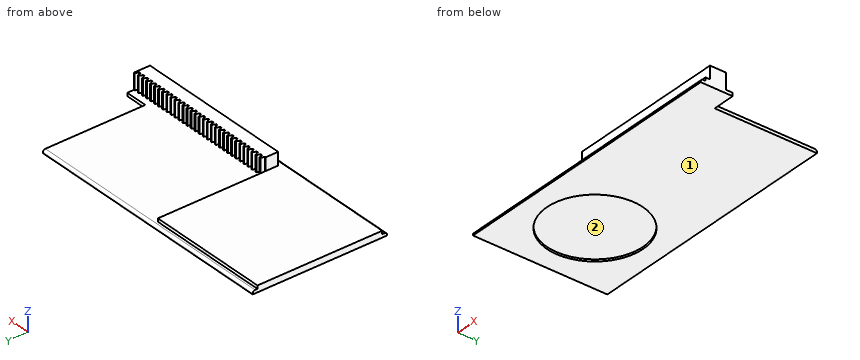
from build123d import *

# Parameters (mm, degrees)
SKETCH1_W           = 206.375
SKETCH1_H           = 106.68
BOSS_EXTRUDE1_DEPTH = 2.54
BOSS_EXTRUDE2_DEPTH = 12.7
SKETCH3_W           = 17.745286293
SKETCH3_H           = 25.4
BOSS_EXTRUDE3_DEPTH = 2.54
FILLET1_R           = 1.905
BOSS_EXTRUDE4_DEPTH = 2.54
SKETCH6_R           = 38.1
CUT_EXTRUDE1_DEPTH  = 1.5875


with BuildPart() as part:
    # Sketch1 → Boss-Extrude1 (new body)
    with BuildSketch(Plane.XY):
        with Locations((49.2125, 0)):
            Rectangle(SKETCH1_W, SKETCH1_H)
    extrude(amount=BOSS_EXTRUDE1_DEPTH)

    # Sketch2 → Boss-Extrude2 (add)
    with BuildSketch(Plane.XY.offset(2.54)):
        Polygon((170.145286293, -33.159030477), (169.379659355, -33.159030477), (168.362726521, -35.953030477), (167.172396462, -35.953030477), (166.155463627, -33.159030477), (165.38983669, -33.159030477), (164.372903855, -35.953030477), (163.182573796, -35.953030477), (162.165640962, -33.159030477), (161.400014024, -33.159030477), (160.38308119, -35.953030477), (159.192751131, -35.953030477), (158.175818296, -33.159030477), (157.410191359, -33.159030477), (156.393258524, -35.953030477), (155.202928465, -35.953030477), (154.185995631, -33.159030477), (153.420368693, -33.159030477), (152.403435859, -35.953030477), (151.2131058, -35.953030477), (150.196172965, -33.159030477), (149.430546028, -33.159030477), (148.413613193, -35.953030477), (147.223283134, -35.953030477), (146.2063503, -33.159030477), (145.440723362, -33.159030477), (144.423790528, -35.953030477), (143.233460469, -35.953030477), (142.216527634, -33.159030477), (141.450900697, -33.159030477), (140.433967862, -35.953030477), (139.243637803, -35.953030477), (138.226704969, -33.159030477), (137.461078031, -33.159030477), (136.444145197, -35.953030477), (135.253815138, -35.953030477), (134.236882303, -33.159030477), (133.471255366, -33.159030477), (132.454322531, -35.953030477), (131.263992472, -35.953030477), (130.247059638, -33.159030477), (129.4814327, -33.159030477), (128.464499866, -35.953030477), (127.274169807, -35.953030477), (126.257236972, -33.159030477), (125.491610035, -33.159030477), (124.4746772, -35.953030477), (123.284347141, -35.953030477), (122.267414307, -33.159030477), (121.501787369, -33.159030477), (120.484854535, -35.953030477), (119.294524476, -35.953030477), (118.277591641, -33.159030477), (117.511964704, -33.159030477), (116.495031869, -35.953030477), (115.30470181, -35.953030477), (114.287768976, -33.159030477), (113.522142038, -33.159030477), (112.505209204, -35.953030477), (111.314879145, -35.953030477), (110.29794631, -33.159030477), (109.532319373, -33.159030477), (108.515386538, -35.953030477), (107.325056479, -35.953030477), (106.308123645, -33.159030477), (105.542496707, -33.159030477), (104.525563873, -35.953030477), (103.335233814, -35.953030477), (102.318300979, -33.159030477), (101.552674042, -33.159030477), (100.535741207, -35.953030477), (99.345411148, -35.953030477), (98.328478314, -33.159030477), (97.562851376, -33.159030477), (96.545918542, -35.953030477), (95.355588483, -35.953030477), (94.338655648, -33.159030477), (93.573028711, -33.159030477), (92.556095876, -35.953030477), (91.365765817, -35.953030477), (90.348832983, -33.159030477), (89.583206045, -33.159030477), (88.566273211, -35.953030477), (87.375943152, -35.953030477), (86.359010317, -33.159030477), (85.59338338, -33.159030477), (84.576450545, -35.953030477), (83.386120486, -35.953030477), (82.369187652, -33.159030477), (81.603560714, -33.159030477), (80.58662788, -35.953030477), (79.396297821, -35.953030477), (78.379364986, -33.159030477), (77.613738049, -33.159030477), (76.596805214, -35.953030477), (75.406475155, -35.953030477), (74.389542321, -33.159030477), (73.623915383, -33.159030477), (72.606982549, -35.953030477), (71.41665249, -35.953030477), (70.399719655, -33.159030477), (69.634092718, -33.159030477), (68.617159883, -35.953030477), (67.426829824, -35.953030477), (66.40989699, -33.159030477), (65.644270052, -33.159030477), (64.627337218, -35.953030477), (63.437007159, -35.953030477), (62.420074324, -33.159030477), (61.654447387, -33.159030477), (60.637514552, -35.953030477), (59.447184493, -35.953030477), (58.430251659, -33.159030477), (57.664624721, -33.159030477), (56.647691887, -35.953030477), (55.457361828, -35.953030477), (54.440428993, -33.159030477), (53.674802056, -33.159030477), (52.657869221, -35.953030477), (51.467539162, -35.953030477), (50.450606328, -33.159030477), (49.68497939, -33.159030477), (48.668046556, -35.953030477), (47.477716497, -35.953030477), (46.460783662, -33.159030477), (45.695156725, -33.159030477), (44.67822389, -35.953030477), (44.083058861, -35.953030477), (44.083058861, -45.979871745), (170.145286293, -45.979871745), align=None)
    extrude(amount=BOSS_EXTRUDE2_DEPTH)

    # Sketch3 → Boss-Extrude3 (add)
    with BuildSketch(Plane(origin=(0, 0, 0), x_dir=(-1, 0, 0), z_dir=(0, 0, -1))):
        with Locations((-161.272643147, -40.64)):
            Rectangle(SKETCH3_W, SKETCH3_H)
    extrude(amount=-BOSS_EXTRUDE3_DEPTH)

    # Fillet1
    fillet1_edges = [part.edges().sort_by_distance(p)[0] for p in [
        (58.085143146, -53.34, 2.54),
        (49.2125, 53.34, 2.54),
    ]]
    fillet(fillet1_edges, radius=FILLET1_R)

    # Sketch5 → Boss-Extrude4 (add)
    with BuildSketch(Plane.XY.offset(2.54)):
        Polygon((-53.975, 49.53), (44.083058861, 49.53), (44.083058861, -45.979871745), (170.145286293, -45.979871745), (170.145286293, -49.53), (44.083058861, -49.53), (-53.975, -49.53), align=None)
    extrude(amount=BOSS_EXTRUDE4_DEPTH)

    # Sketch6 → Cut-Extrude1 (cut)
    with BuildSketch(Plane(origin=(0, 0, 0), x_dir=(-1, 0, 0), z_dir=(0, 0, -1))):
        Circle(SKETCH6_R)
    extrude(amount=-CUT_EXTRUDE1_DEPTH, mode=Mode.SUBTRACT)


solid = part.part
Verification items for the finished model (mm, model axes). Face numbers are marked on the shaded views. Give positions to 0.01 mm unless a question says otherwise; leave off trailing zeros. Write each loop counter-clockwise with the first axis right and the second up, starting at its lowest first coordinate (ties: lowest second). Pieces come first, ordered by that corner, then holes. Notation, with made-up numbers: (80, -16.75) - (94, -16.75) arc R35 ccw to (94, 17.25) - close; hole circle Ø6 at (-27, 23.25). An arc over 180 degrees is marked (long way). Answer as CSV lines item,"result". Start each with the question number.
1. Sectioned sample at D-D (y = -8). Record the boundary of the cut face in (x, z) (1 decimal), then the cut area to 3 significant figures.
2. Sectioned sample at B-B (y = -41.5). Record the boundary of the cut face in (x, z) (3 decimals), then the cut area to 3 significant figures.
3. Depth check by flat-ended pin: pin 1 (0.8 mm diameter, centred on x = 169.5, z = 6.5, fed in from +Y); pin 2 (1 mm diameter, centred on y = 0.5, z = 4, fed in from +X); pin 3 (0.6 mm diameter, centred on x = 96, z = 8.5, fed in from +Y). Enter the tip coordinate at first touch or a pass-through.
4. Draft check along Y on the marked faces 1 and 2. Enter one of: pulls with the +Y half, pulls with the -Y half, needs draft (parallel to the pull), parting line crosses it, or undercut.
5. Sectioned sample at A-A (x = 0). Record the boundary of the cut face in (y, z) (1 decimal), then the cut area to 3 significant figures.
6. Sectioned sample at C-C (y = 20). Record the boundary of the cut face in (x, z) (1 decimal).
7. Thickness scan on line 1 (Y direction, x = 0, z = 0.55); line 2 (X direction, y = -42.5, z = 5.5); line 3 (Z direction, x = 107, y = 39.5). Record the ranges inside material, lowest first.
Derived:
1,outline,"(-54, 0) - (-37.3, 0) - (-37.3, 1.6) - (37.3, 1.6) - (37.3, 0) - (152.4, 0) - (152.4, 2.5) - (44.1, 2.5) - (44.1, 5.1) - (-54, 5.1) - close"
1,area,"655 mm²"
2,outline,"(-53.975, 0) - (170.145, 0) - (170.145, 15.24) - (44.083, 15.24) - (44.083, 5.08) - (-53.975, 5.08) - close"
2,area,"2,420 mm²"
3,pin 1,"y = -33.16"
3,pin 2,"x = 44.08"
3,pin 3,"y = -35.95"
4,face 1,"needs draft"
4,face 2,"undercut"
5,outline,"(-53.3, 0) - (-38.1, 0) - (-38.1, 1.6) - (38.1, 1.6) - (38.1, 0) - (53.3, 0) - (53.3, 0.6) arc R1.9 ccw to (51.4, 2.5) - (49.5, 2.5) - (49.5, 5.1) - (-49.5, 5.1) - (-49.5, 2.5) - (-51.4, 2.5) arc R1.9 ccw to (-53.3, 0.6) - close"
5,area,"400 mm²"
6,outline,"(-54, 0) - (-32.4, 0) - (-32.4, 1.6) - (32.4, 1.6) - (32.4, 0) - (152.4, 0) - (152.4, 2.5) - (44.1, 2.5) - (44.1, 5.1) - (-54, 5.1) - close"
7,line 1,"-53.34 to -38.1, 38.1 to 53.34"
7,line 2,"44.08 to 170.15"
7,line 3,"0 to 2.54"
